Geometry: see drawing. Coordinates: mm, zero at the bounding-box minimum. A direction names the side the tool comes from. Coordinates: 2 decimals unless noted, no trailing zeros. Order: outer loops, then holes, each group sorted by start corner. A loop starts at its lowest first (then second) coordinate and runs counter-clockwise, first axis right, second up.
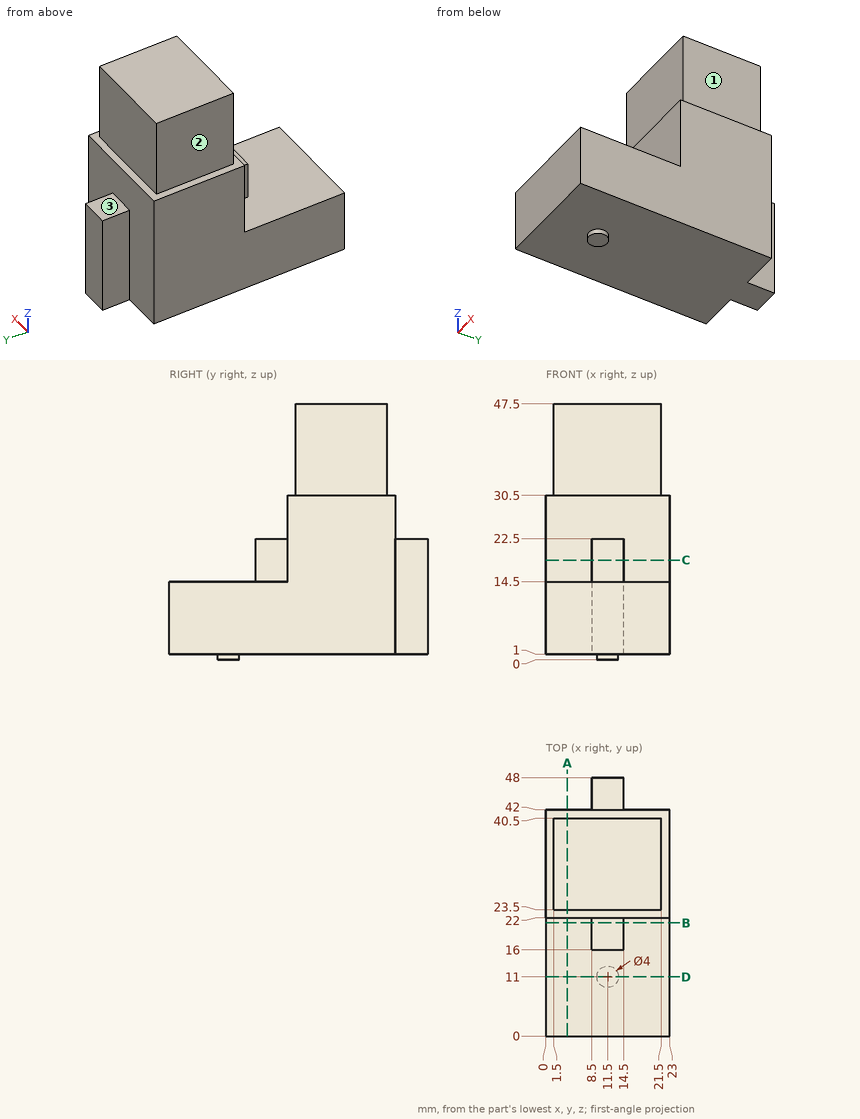
Item 1: Cut plane D-D on y = 11. Return loops of the section in (x, z), then the cut area to 4 significant figures.
Response values:
outline: (0, 1) - (9.5, 1) - (9.5, 0) - (13.5, 0) - (13.5, 1) - (23, 1) - (23, 14.5) - (0, 14.5) - close
area: 314.5 mm2
Item 2: Cut plane B-B on y = 21. Return loops of the section in (x, z).
Response values:
outline: (0, 1) - (23, 1) - (23, 14.5) - (14.5, 14.5) - (14.5, 22.5) - (8.5, 22.5) - (8.5, 14.5) - (0, 14.5) - close
Item 3: Cut plane C-C on z = 18.5. Return loops of the section in (x, y), then the cut area to 3 significant figures.
Response values:
outline: (0, 22) - (8.5, 22) - (8.5, 16) - (14.5, 16) - (14.5, 22) - (23, 22) - (23, 42) - (14.5, 42) - (14.5, 48) - (8.5, 48) - (8.5, 42) - (0, 42) - close
area: 532 mm2
Item 4: Pin query (flat end, axial travel): pin 1 Ø3 at (y, z) = (20, 17) entering from +X; pin 2 Ø7 at (x, y) = (10.5, 30.5) entering from -Z; pin 3 Ø12 at (y, z) = (40, 37) entering from +X; pin 4 Ø10 at (x, z) = (4, 5.5) entering from -Y. Return the tip coordinate at first contact, or that it passes through.
Response values:
pin 1: stops at x = 14.5
pin 2: stops at z = 1
pin 3: stops at x = 21.5
pin 4: stops at y = 0
Item 5: Ray query, probe 1 along X at (y, z) = (35, 38); probe 2 along Z at (x, y) = (4, 13); probe 3 along Y at (x, z) = (15.75, 28.5). Return the intervals inside material, ascending.
Response values:
probe 1: x = 1.5 to 21.5
probe 2: z = 1 to 14.5
probe 3: y = 22 to 42
Item 6: Cut plane A-A on x = 4. Return loops of the section in (y, z), then the cut area to 3 significant figures.
Response values:
outline: (0, 1) - (42, 1) - (42, 30.5) - (40.5, 30.5) - (40.5, 47.5) - (23.5, 47.5) - (23.5, 30.5) - (22, 30.5) - (22, 14.5) - (0, 14.5) - close
area: 1,180 mm2
Item 7: Access query for the marked faces 1, 2 and 3. Directions: +Z, -Z, +X, -X, +Y, -Y. A direction counts if a zero-diameter tool reaches every point of the face in a straight line with its end or side. Return the directions, or none.
Response values:
face 1: +Z, +X, +Y, -Y
face 2: +Z, -X, +Y, -Y
face 3: +Z, +X, -X, +Y
